Can you work these out from the model? Positions are in its coordinate system, mm. A direction names the side the tool comes from. Round coordinates to 2 decimals unless told otherwise and drop trailing zeros. Loops run counter-clockwise (first coordinate to the right, second up) from the corner with the lowest first, then second, coordinate; pieces in that order, holes last. Notation, with made-up numbers: M -10.75,76.5 L 19.25,76.5 A20 ccw 19.25,96.5 Z; hole C -0.5,25.25 d8. An arc over 180 degrees is marked long. Use a Markdown table: item, result. Add a question column.
```python
from build123d import *

# Parameters (mm, degrees)
SM_BASE_FLANGE_1_DEPTH = 491
CUT_EXTRUDE_1_REACH    = 576.223
CUT_EXTRUDE_2_DEPTH    = 575.223290751
PATTERN_LINEAR_1_COUNT = 4
PATTERN_LINEAR_1_PITCH = 50
FILLET_1_R             = 30
SKETCH_4_W             = 685
SKETCH_4_H             = 100
EXTRUDE_1_DEPTH        = 10
CUT_EXTRUDE_3_DEPTH    = 10
FILLET_2_R             = 10


# Sheet-metal steps are written as plain solids
with BuildPart() as part:
    # Sketch 1 → 基体-法兰1 (new, symmetric)
    with BuildSketch(Plane(origin=(0, 0, 0), x_dir=(0, 0, -1), z_dir=(1, 0, 0))):
        with BuildLine():
            Line((0, 0), (230, 0))
            ThreePointArc((230, 0), (237.071067812, 2.928932188), (240, 10))
            Line((240, 10), (240, 106.074175964))
            ThreePointArc((240, 106.074175964), (239.819563867, 107.965251176), (239.284766909, 109.788082728))
            Line((239.284766909, 109.788082728), (220, 158))
            Line((220, 158), (229.284766909, 161.713906764))
            Line((229.284766909, 161.713906764), (248.569533818, 113.501989491))
            ThreePointArc((248.569533818, 113.501989491), (249.639127735, 109.856326387), (250, 106.074175964))
            Line((250, 106.074175964), (250, 10))
            ThreePointArc((250, 10), (244.142135624, -4.142135624), (230, -10))
            Line((230, -10), (0, -10))
            Line((0, -10), (0, 0))
        make_face()
    extrude(amount=SM_BASE_FLANGE_1_DEPTH, both=True)

    # Sketch 2 → 切除-拉伸1 (cut, up to next)
    with BuildSketch(Plane(origin=(0, 0, -250), x_dir=(-1, 0, 0), z_dir=(0, 0, -1)), mode=Mode.PRIVATE) as cut_extrude_1_sk1:
        Polygon((-411, 161.713906764), (-411, 82), (-491, 62), (-491, 161.713906764), align=None)
    cut_extrude_1_tool1 = extrude(cut_extrude_1_sk1.sketch, amount=-CUT_EXTRUDE_1_REACH, mode=Mode.PRIVATE) & part.part
    # Sketch 2 → 切除-拉伸1 (cut, up to next)
    with BuildSketch(Plane(origin=(0, 0, -250), x_dir=(-1, 0, 0), z_dir=(0, 0, -1)), mode=Mode.PRIVATE) as cut_extrude_1_sk2:
        Polygon((491, 161.713906764), (411, 161.713906764), (411, 82), (491, 62), align=None)
    cut_extrude_1_tool2 = extrude(cut_extrude_1_sk2.sketch, amount=-CUT_EXTRUDE_1_REACH, mode=Mode.PRIVATE) & part.part
    add(cut_extrude_1_tool1.solids().sort_by_distance((452.486206, 116.671178, -250))[0], mode=Mode.SUBTRACT)
    add(cut_extrude_1_tool2.solids().sort_by_distance((-452.486206, 116.671178, -250))[0], mode=Mode.SUBTRACT)

    # 草图3 → 切除-拉伸2 (cut, through all)
    with BuildSketch(Plane(origin=(0, 0, 0), x_dir=(1, 0, 0), z_dir=(0, 1, 0))):
        with BuildLine():
            Line((466, 57.5), (471, 57.5))
            ThreePointArc((471, 57.5), (478.5, 50), (471, 42.5))
            Line((471, 42.5), (466, 42.5))
            ThreePointArc((466, 42.5), (458.5, 50), (466, 57.5))
        make_face()
        with BuildLine():
            Line((-466, 42.5), (-471, 42.5))
            ThreePointArc((-471, 42.5), (-478.5, 50), (-471, 57.5))
            Line((-471, 57.5), (-466, 57.5))
            ThreePointArc((-466, 57.5), (-458.5, 50), (-466, 42.5))
        make_face()
    cut_extrude_2 = extrude(amount=-CUT_EXTRUDE_2_DEPTH, mode=Mode.SUBTRACT)

    # 阵列(线性)1: 切除-拉伸2 ×4
    with Locations(*[(0, 0, -i * PATTERN_LINEAR_1_PITCH) for i in range(1, PATTERN_LINEAR_1_COUNT)]):
        add(cut_extrude_2, mode=Mode.SUBTRACT)

    # 圆角1
    fillet_1_edges = [part.edges().sort_by_distance(p)[0] for p in [
        (411, 159.856953382, -224.642383454),
        (-411, 159.856953382, -224.642383454),
    ]]
    fillet(fillet_1_edges, radius=FILLET_1_R)

    # 草图4 → 凸台-拉伸1 (add)
    with BuildSketch(Plane(origin=(0, 0, 0), x_dir=(1, 0, 0), z_dir=(0, 1, 0))):
        with Locations((0, -50)):
            Rectangle(SKETCH_4_W, SKETCH_4_H)
    extrude(amount=-EXTRUDE_1_DEPTH)

    # 草图5 → 切除-拉伸3 (cut)
    with BuildSketch(Plane(origin=(0, 0, 0), x_dir=(1, 0, 0), z_dir=(0, 1, 0))):
        with BuildLine():
            Line((-31.5, -47.5), (-31.5, -52.5))
            ThreePointArc((-31.5, -52.5), (-40, -61), (-48.5, -52.5))
            Line((-48.5, -52.5), (-48.5, -47.5))
            ThreePointArc((-48.5, -47.5), (-40, -39), (-31.5, -47.5))
        make_face()
        with BuildLine():
            Line((48.5, -47.5), (48.5, -52.5))
            ThreePointArc((48.5, -52.5), (40, -61), (31.5, -52.5))
            Line((31.5, -52.5), (31.5, -47.5))
            ThreePointArc((31.5, -47.5), (40, -39), (48.5, -47.5))
        make_face()
    extrude(amount=-CUT_EXTRUDE_3_DEPTH, mode=Mode.SUBTRACT)

    # 圆角2
    fillet_2_edges = [part.edges().sort_by_distance(p)[0] for p in [
        (491, 62, -245),
        (411, 82, -245),
        (-411, 82, -245),
        (-491, 62, -245),
    ]]
    fillet(fillet_2_edges, radius=FILLET_2_R)


solid = part.part
```
(1) Suppose I cut it at D-D on x = 266. List the corners of the cut face in (y, z) for me.
(2) If I drill on probe 1 along Z at (x, y) = (-395, 9); probe 2 along Y at (x, z) = (415.5, -8); probe 3 along Z at (x, y) = (124.5, 73), over which ranges is the centre line in solid material (lowest first)? Write a range as [from, to].
(3) I'm going to push flat-ended pins straight in: pin 1 (1.5 mm diameter, centred on x = 469.5, y = -3.5, fed in from -Z); pin 2 (15 mm diameter, centred on y = 104, z = -238.5, fed in from +X); pin 3 (5.5 mm diameter, centred on x = 469.5, y = -7.5, fed in from -Z). Where does each tip first touch, or does it pass through?
(4) Suppose I cut it at C-C on z = -13. List the corners of the cut face in (x, y) for me, and give its area (3 significant figures).
(5) On a 3-axis mill with a long thin cutter (end or side, diameter ignored), from which of +Z, -Z, +X, -X, +Y, -Y can I reach the whole of each face in a straight line? I mean faces 1 (the face through (411, 112, -243)), 2 (the face through (-411, 112, -243)), 3 (the face through (7, 57, -240)). Say none if no direction works.
(6) Suppose I cut it at B-B on x = -369. List the corners of the cut face in (y, z) for me.
(7) Suppose I cut it at A-A on x = 40. List the corners of the cut face in (y, z) for me, and give its area (3 significant figures).
Results below:
| question | item | result |
|---|---|---|
| 1 | outline | M -10,-230 A20 ccw 10,-250 L 106.07,-250 A20 ccw 113.5,-248.57 L 161.71,-229.28 L 158,-220 L 109.79,-239.28 A10 cw 106.07,-240 L 10,-240 A10 cw 0,-230 L 0,100 L -10,100 Z |
| 2 | probe 1 | z = [-249.97, -239.95] |
| 2 | probe 2 | y = [-10, 0] |
| 2 | probe 3 | z = [-250, -240] |
| 3 | pin 1 | stops at z = -245.41 |
| 3 | pin 2 | stops at x = 411 |
| 3 | pin 3 | stops at z = -243.51 |
| 4 | outline | M -491,-10 L 491,-10 L 491,0 L -491,0 Z |
| 4 | area | 9,820 mm² |
| 5 | face 1 | +Z, -Z, +X, +Y |
| 5 | face 2 | +Z, -Z, -X, +Y |
| 5 | face 3 | +Z, +X, -X |
| 6 | outline | M -10,-230 A20 ccw 10,-250 L 106.07,-250 A20 ccw 113.5,-248.57 L 161.71,-229.28 L 158,-220 L 109.79,-239.28 A10 cw 106.07,-240 L 10,-240 A10 cw 0,-230 L 0,0 L -10,0 Z |
| 7 | outline | M -10,-230 A20 ccw 10,-250 L 106.07,-250 A20 ccw 113.5,-248.57 L 161.71,-229.28 L 158,-220 L 109.79,-239.28 A10 cw 106.07,-240 L 10,-240 A10 cw 0,-230 L 0,39 L -10,39 Z; M -10,61 L 0,61 L 0,100 L -10,100 Z |
| 7 | area | 4,850 mm² |
